Work out the finished part from the listing and answer in its coordinate system (mm). Face numbers are marked on the shaded views. Round coordinates to 2 decimals unless told otherwise and drop trailing zeros. Loops run counter-clockwise (first coordinate to the right, second up) from the corner with the lowest first, then second, coordinate; pieces in that order, holes last. Notation, with made-up numbers: (50.5, 21) -> (108.5, 21) arc R31 cw to (108.5, 58) -> close; hole circle Ø1 at (52, -20). An arc over 180 degrees is marked (long way). Use one line per item in the form item = value.
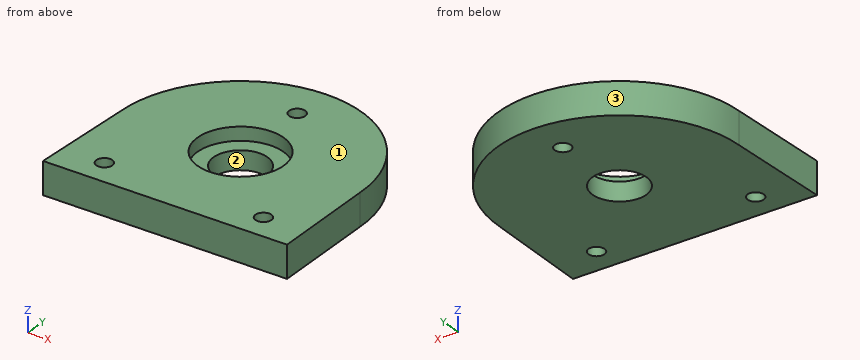
```python
from build123d import *

# Parameters (mm, degrees)
BEARING_HOLDER_BOSS_EXTRUDE1_DEPTH = 6
SKETCH2_R                          = 8
BEARING_HOLE_CUT_EXTRUDE1_DEPTH    = 2.5
SKETCH3_R                          = 5
SHAFT_HOLE_CUT_EXTRUDE2_DEPTH      = 3.5
SKETCH4_R                          = 1.5
MOUNTING_HOLES_CUT_EXTRUDE3_DEPTH  = 6


with BuildPart() as part:
    # Sketch1 → Bearing Holder Boss-Extrude1 (new body)
    with BuildSketch(Plane.XY):
        with BuildLine():
            Line((-22.5, 0), (-22.999267837, -20))
            Line((-22.999267837, -20), (0, -20))
            Line((0, -20), (22.999267837, -20))
            Line((22.999267837, -20), (22.5, 0))
            ThreePointArc((22.5, 0), (0, 22.5), (-22.5, 0))
        make_face()
    extrude(amount=-BEARING_HOLDER_BOSS_EXTRUDE1_DEPTH)

    # Sketch2 → Bearing Hole Cut-Extrude1 (cut)
    with BuildSketch(Plane.XY):
        Circle(SKETCH2_R)
    extrude(amount=-BEARING_HOLE_CUT_EXTRUDE1_DEPTH, mode=Mode.SUBTRACT)

    # Sketch3 → Shaft Hole Cut-Extrude2 (cut)
    with BuildSketch(Plane.XY.offset(-2.5)):
        Circle(SKETCH3_R)
    extrude(amount=-SHAFT_HOLE_CUT_EXTRUDE2_DEPTH, mode=Mode.SUBTRACT)

    # Sketch4 → Mounting Holes Cut-Extrude3 (cut)
    with BuildSketch(Plane.XY):
        with Locations((0, 15)):
            Circle(SKETCH4_R)
        with Locations((-15, -15)):
            Circle(SKETCH4_R)
        with Locations((15, -15)):
            Circle(SKETCH4_R)
    extrude(amount=-MOUNTING_HOLES_CUT_EXTRUDE3_DEPTH, mode=Mode.SUBTRACT)


solid = part.part
```
(1) For a pull along X with two mould halves and no side action, classify the marked faces 1, 2 and 3 as +X half, -X half, draft (parallel to the pull), parting line (faces both ways), or undercut.
Completed:
face_1 = draft
face_2 = undercut
face_3 = parting line
(2) Find section B-B, the plane x = -4. Write down the section's boundary in (y, z).
Completed:
outline = (-20, -6) -> (-3, -6) -> (-3, -2.5) -> (-6.93, -2.5) -> (-6.93, 0) -> (-20, 0) -> close; (3, -6) -> (22.14, -6) -> (22.14, 0) -> (6.93, 0) -> (6.93, -2.5) -> (3, -2.5) -> close
(3) Find section D-D, the plane y = -6.5. Write down the section's boundary in (x, z), then the cut area to 3 significant figures.
Completed:
outline = (-22.66, -6) -> (22.66, -6) -> (22.66, 0) -> (4.66, 0) -> (4.66, -2.5) -> (-4.66, -2.5) -> (-4.66, 0) -> (-22.66, 0) -> close
area = 249 mm2
(4) Consider L1, parallel to Y at x = 0, z = -1.95; L2, parallel to Y at x = 0, z = -3.95; L3, parallel to Y at x = -15, z = -4. Determine where each line is inside the solid, lowest interval first.
Completed:
L1 = -20 to -8, 8 to 13.5, 16.5 to 22.5
L2 = -20 to -5, 5 to 13.5, 16.5 to 22.5
L3 = -20 to -16.5, -13.5 to 16.77
(5) Find section A-A, the plane y = 15. Write down the section's boundary in (x, z), then the cut area to 3 significant figures.
Completed:
outline = (-16.77, -6) -> (-1.5, -6) -> (-1.5, 0) -> (-16.77, 0) -> close; (1.5, -6) -> (16.77, -6) -> (16.77, 0) -> (1.5, 0) -> close
area = 183 mm2
(6) Find section C-C, the plane y = -1.5. Write down the section's boundary in (x, z), then the cut area to 3 significant figures.
Completed:
outline = (-22.54, -6) -> (-4.77, -6) -> (-4.77, -2.5) -> (-7.86, -2.5) -> (-7.86, 0) -> (-22.54, 0) -> close; (4.77, -6) -> (22.54, -6) -> (22.54, 0) -> (7.86, 0) -> (7.86, -2.5) -> (4.77, -2.5) -> close
area = 198 mm2
(7) Given P1, Ø17.5, axis at x = -1.5, y = 4, coming from the +Z side; P2, Ø1.5, axis at y = 3.5, z = -3, coming from the +X side; P3, Ø2.5, axis at x = 0, y = 15, coming from the +Z side, each flat-ended and moving along its own axis, determine where each tip first touches the part or whether it passes through.
Completed:
P1 = 0
P2 = 22.33
P3 = through
